Read the model definition and answer for the solid it produces. Units are mm, in the model's axes. A direction names the side the tool comes from. Round coordinates to 2 decimals unless told otherwise and drop trailing zeros. Order: outer loops, then holes, each group sorted by start corner. A loop starts at its lowest first (then second) coordinate and runs counter-clockwise, first axis right, second up.
from build123d import *

# Parameters (mm, degrees)
BOSS_EXTRUDE1_DEPTH                             = 12.7
SKETCH2_R                                       = 9.525
SKETCH3_R                                       = 6.985
FILLET1_R                                       = 0.254
CUT_EXTRUDE1_DEPTH                              = 2.54
CUT_EXTRUDE1_DEPTH_BACK                         = 19.412260753
SKETCH4_R                                       = 2.286
SCALE1_SCALE                                    = 1.5
CBORE_FOR_1_PAN_HEAD_MACHINE_SCREW2_D           = 2.0574
CBORE_FOR_1_PAN_HEAD_MACHINE_SCREW2_CBORE_D     = 4.36626
CBORE_FOR_1_PAN_HEAD_MACHINE_SCREW2_CBORE_DEPTH = 0.508


with BuildPart() as part:
    # Sketch1 → Boss-Extrude1 (new body)
    with BuildSketch(Plane.XY):
        with BuildLine():
            ThreePointArc((5.819871133, 2.54), (0, 6.35), (-5.819871133, 2.54))
            Line((-5.819871133, 2.54), (-3.81, 2.54))
            Line((-3.81, 2.54), (-3.81, -2.54))
            Line((-3.81, -2.54), (-5.819871133, -2.54))
            ThreePointArc((-5.819871133, -2.54), (0, -6.35), (5.819871133, -2.54))
            Line((5.819871133, -2.54), (3.81, -2.54))
            Line((3.81, -2.54), (3.81, 2.54))
            Line((3.81, 2.54), (5.819871133, 2.54))
        make_face()
    extrude(amount=BOSS_EXTRUDE1_DEPTH)

    # Sketch2 → Loft1 section 0
    with BuildSketch(Plane(origin=(0, 0, 0), x_dir=(-1, 0, 0), z_dir=(0, 0, -1))):
        Circle(SKETCH2_R)
    # Sketch3 → Loft1 section 1
    with BuildSketch(Plane.XY.offset(-7.62)):
        Circle(SKETCH3_R)
    loft()

    # Fillet1
    fillet1_edges = [part.edges().sort_by_distance(p)[0] for p in [
        (9.525, 0, 0),
        (6.985, 0, -7.62),
    ]]
    fillet(fillet1_edges, radius=FILLET1_R)

    # Sketch4 → Cut-Extrude1 (cut, two sides: drawn at the far end of the back side and taken through both)
    with BuildSketch(Plane(origin=(0, 0, 0), x_dir=(1, 0, 0), z_dir=(0, 1, 0)).offset(-CUT_EXTRUDE1_DEPTH_BACK)):
        with Locations(Location((0, -6.35, 0), (0, 0, 90))):
            Circle(SKETCH4_R)
    extrude(amount=CUT_EXTRUDE1_DEPTH + CUT_EXTRUDE1_DEPTH_BACK, mode=Mode.SUBTRACT)


with BuildPart() as part_1:
    # Scale1: scaled about (5.44e-07, 0.095418274, 0.619819033)
    add(part.part.scale(SCALE1_SCALE).moved(Location((-2.72e-07, -0.047709137, -0.309909516))))

    # CBORE for #1 Pan Head Machine Screw2 (through all)
    with Locations(Plane(origin=(5.715002511, 0, 0), x_dir=(0, 0, -1), z_dir=(1, 0, 0))):
        with Locations((-9.2150808, -0.047706209)):
            cbore_for_1_pan_head_machine_screw2 = CounterBoreHole(CBORE_FOR_1_PAN_HEAD_MACHINE_SCREW2_D / 2, CBORE_FOR_1_PAN_HEAD_MACHINE_SCREW2_CBORE_D / 2, CBORE_FOR_1_PAN_HEAD_MACHINE_SCREW2_CBORE_DEPTH)

    # Mirror1: CBORE for #1 Pan Head Machine Screw2 across plane
    add(cbore_for_1_pan_head_machine_screw2.mirror(Plane(origin=(0, 0, 0), x_dir=(0, 0, 1), z_dir=(1, 0, 0))), mode=Mode.SUBTRACT)


solid = part_1.part
Q1. Straight lines are drawn through the part: probe 1 along Z at (x, y) = (0, -0.5); probe 2 along Z at (x, y) = (8, 0.5); probe 3 along X at (y, z) = (-7.5, 8.5). For each, find the intervals that lie inside material, in ascending order.
Outcome:
probe 1: z = -11.74 to 5.79, 12.64 to 18.74
probe 2: z = -11.74 to -0.31
probe 3: x = -5.93 to -3.35, 3.35 to 5.93
Q2. A cutting plane is placed at A-A, the plane z = -6. Give the vertices of the cut face in (x, y).
Outcome:
outline: circle Ø24.78 at (0, -0.05)
Q3. For a pull along Y with two mould halves and no side action, classify faces 6 (the face through (5.715, -1, 7)), 7 (the face through (-0.15, -9.57, 4.85)), 8 (the face through (5.465, 0.608, 7.133)), 9 (the face through (2.413, -10.915, -9.776)) as released by +Y, released by -Y, zero draft, split by the parting line, or undercut.
Outcome:
face 6: undercut
face 7: released by -Y
face 8: undercut
face 9: split by the parting line
Q4. For faces 1 (the face through (-5.715, 1, 7)), 2 (the face through (-5.465, 0.608, 7.133)), 3 (the face through (1.313, -3.002, 6.048)), 4 (the face through (0.155, 9.476, 9.082)), 5 (the face through (7, -3.858, 9)), determine the directions among +Z, -Z, +X, -X, +Y, -Y from which every point of the face is accessible in a straight line to the end or side of a thin tool.
Outcome:
face 1: +Z, -X
face 2: -X
face 3: -Y
face 4: +Z, +Y
face 5: +Z, +X
Q5. Flat-ended cylindrical pins translate along their axes: pin 1 (3.5 mm diameter, centred on y = -0.5, z = 8.5, fed in from +X) (3 decimals); pin 2 (5 mm diameter, centred on x = -8.5, z = 12.5, fed in from -Y); pin 3 (1 mm diameter, centred on y = -5, z = 1.5, fed in from +X). Find the tip coordinate at first contact, or state that the pin passes through.
Outcome:
pin 1: stops at x = 5.715
pin 2: stops at y = -7.45
pin 3: stops at x = 8.42
